Read the model definition and answer for the solid it produces. Units are mm, in the model's axes. A direction names the side the tool comes from. Give positions to 0.01 mm unless a question says otherwise; leave off trailing zeros. Write each loop counter-clockwise with the first axis right and the second up, starting at its lowest first coordinate (ties: lowest second). Pieces come first, ordered by that corner, then holes. Notation, with made-up numbers: (74.25, 60.25) -> (125.25, 60.25) arc R9 cw to (125.25, 66.25) -> close; hole circle Ø8 at (-21.75, 53.5). An arc over 180 degrees is marked (long way). Write item = value, one per line.
from build123d import *

# Parameters (mm, degrees)
BOSS_EXTRU_1_DEPTH = 10
ESQUISSE2_R        = 10
BOSS_EXTRU_2_DEPTH = 20


with BuildPart() as part:
    # Esquisse1 → Boss.-Extru.1 (new body)
    with BuildSketch(Plane.XY):
        with BuildLine():
            Line((-30, 0), (30, 0))
            Line((30, 0), (30, 20))
            Line((30, 20), (20, 20))
            Line((20, 20), (20, 40))
            ThreePointArc((20, 40), (0, 60), (-20, 40))
            Line((-20, 40), (-20, 20))
            Line((-20, 20), (-30, 20))
            Line((-30, 20), (-30, 0))
        make_face()
    extrude(amount=BOSS_EXTRU_1_DEPTH)

    # Esquisse2 → Boss.-Extru.2 (add)
    with BuildSketch(Plane.XY.offset(10)):
        with Locations((0, 40)):
            Circle(ESQUISSE2_R)
    extrude(amount=BOSS_EXTRU_2_DEPTH)


solid = part.part
(1) The part is cut by section A-A on x = 0. Determine the outline of the cut face in (y, z), plus the area to 3 significant figures.
Checks:
outline = (0, 0) -> (60, 0) -> (60, 10) -> (50, 10) -> (50, 30) -> (30, 30) -> (30, 10) -> (0, 10) -> close
area = 1,000 mm²
(2) The part is cut by section C-C on z = 26. Determine the outline of the cut face in (x, y), plus the area to 3 significant figures.
Checks:
outline = circle Ø20 at (0, 40)
area = 314 mm²
(3) The part is cut by section D-D on x = -23. Determine the outline of the cut face in (y, z), plus the area to 3 significant figures.
Checks:
outline = (0, 0) -> (20, 0) -> (20, 10) -> (0, 10) -> close
area = 200 mm²
(4) Given P1, Ø12, axis at x = -5.5, z = 6, coming from the +Y side; P2, Ø11, axis at y = 29.5, z = 4, coming from the +X side; P3, Ø8, axis at y = 25.5, z = 5.5, coming from the -X side, each flat-ended and moving along its own axis, determine where each tip first touches the part or whether it passes through.
Checks:
P1 = 60
P2 = 20
P3 = -20
(5) A tool of negligible diameter and unlimited length cuts with its end or side. For faces 1 (the flat face through (25, 20, 5)), 2 (the flat face through (-25, 20, 5)), 3 (the cylindrical face through (-2.17, 30.24, 19.86)), from which of +Z, -Z, +X, -X, +Y, -Y can it reach the whole face along a straight path? Write none if from no direction.
Checks:
face_1 = +Z, -Z, +X, +Y
face_2 = +Z, -Z, -X, +Y
face_3 = +Z
(6) The part is cut by section B-B on y = 39. Determine the outline of the cut face in (x, z), plus the area to 3 significant figures.
Checks:
outline = (-20, 0) -> (20, 0) -> (20, 10) -> (9.95, 10) -> (9.95, 30) -> (-9.95, 30) -> (-9.95, 10) -> (-20, 10) -> close
area = 798 mm²
(7) Consider L1, parallel to Y at x = 23, z = 7.25; L2, parallel to Z at x = -11.5, y = 29; L3, parallel to X at y = 29, z = 3.5. Determine where each line is inside the solid, lowest interval first.
Checks:
L1 = 0 to 20
L2 = 0 to 10
L3 = -20 to 20
